Source: CAD feature listing. Evaluate the final solid. Frame: model axes, mm. Face numbers are marked on the shaded views. A direction names the side the tool comes from. Give positions to 0.01 mm unless a question says otherwise; leave off trailing zeros. Write each loop counter-clockwise with the first axis right and the second up, starting at its lowest first coordinate (ties: lowest second). Pieces come first, ordered by that corner, then holes. Notation, with made-up numbers: M 20.25,-10 L 34.25,-10 A19 cw 34.25,10 Z; hole C -10,78.5 d9. An arc over 180 degrees is marked long. Return JSON: item names as keys, results as strings.
Autodesk Inventor part; units mm, degrees
ref_plane "YZ Plane" through (0, 0, 0) normal (1, 0, 0) x (0, 1, 0)
ref_plane "XZ Plane" through (0, 0, 0) normal (0, 1, 0) x (-1, 0, 0)
ref_plane "XY Plane" through (0, 0, 0) normal (0, 0, 1) x (1, 0, 0)
sketch "Sketch1" plane through (0, 0, 0) normal (0, 1, 0) x (-1, 0, 0)
  point P0 (0, 0)
sketch "Sketch2" plane through (0, 0, 0) normal (0, 1, 0) x (-1, 0, 0)
  line L0 (68, -12) -> (68, -66)
  line L1 (68, -66) -> (0, -66)
  line L2 (0, -66) -> (0, -12)
  line L3 (68, -12) -> (0, -12)
  point P0 (0, 0)
  dimension "d0" = 68
  dimension "d138" = 54
extrude "Extrusion1" add sketch "Sketch2" along normal blind 14
sketch "Sketch3" plane through (0, 14, 0) normal (0, 1, 0) x (1, 0, 0)
  point P0 (-68, 66)
sketch "Sketch4" plane through (0, 14, 0) normal (0, 1, 0) x (1, 0, 0)
  line L0 (0, 66) -> (-68, 66)
  line L1 (-30.4814, 66) -> (-28.4814, 66)
  line L2 (-28.4814, 66) -> (-28.4814, 64)
  line L3 (-68, 66) -> (-68, 12)
  line L4 (-68, 37.8423) -> (-68, 39.8423)
  line L5 (-68, 39.8423) -> (-66, 39.8423)
  line L6 (0, 38.8423) -> (0, 36.8423)
  line L7 (0, 36.8423) -> (-2, 36.8423)
  line L8 (-66, 64) -> (-2, 64)
  line L9 (-2, 64) -> (-2, 14)
  line L10 (-2, 14) -> (-66, 14)
  line L11 (-66, 14) -> (-66, 64)
  dimension "d5" = 2
  dimension "d6" = 2
  dimension "d7" = 2
  dimension "d11" = 2
  dimension "d75" = 2
  dimension "d132" = 50
  dimension "d133" = 64
extrude "Extrusion2" cut sketch "Sketch4" against normal blind 13 contours L8 L9 L10 L11
sketch "Sketch7" plane through (0, 14, 0) normal (0, 1, 0) x (1, 0, 0)
  line L0 (-68, 66) -> (-67, 66)
  line L1 (-68, 66) -> (-6, 66)
  line L2 (-68, 65) -> (-68, 66)
  line L3 (0, 66) -> (-7, 66)
  line L4 (-67, 65) -> (-1, 65)
  line L5 (0, 66) -> (-68, 66)
  line L6 (-68, 66) -> (0, 66)
  line L7 (0, 12) -> (0, 66)
  line L8 (0, 12) -> (-1, 12)
  line L9 (-1, 66) -> (0, 66)
  line L10 (0, 66) -> (0, 12)
  line L11 (0, 12) -> (-1, 12)
  line L12 (-68, 12) -> (0, 12)
  line L13 (-1, 65) -> (-1, 12)
  line L14 (0, 12) -> (-1, 12)
  line L15 (-67, 65) -> (-67, 12)
  line L16 (-68, 66) -> (-68, 12)
  line L17 (-67, 12) -> (-68, 12)
  line L18 (-68, 12) -> (-68, 66)
  dimension "d76" = 1
  dimension "d139" = 1
  dimension "d140" = 1
extrude "Extrusion3" cut sketch "Sketch7" against normal blind 2 contours L0 L1 L3 L7 L8 L13 L4 L15 L12 L16 L2
sketch "Sketch8" plane through (0, 14, 0) normal (0, 1, 0) x (1, 0, 0)
  line L0 (0, 12) -> (0, 13)
  line L1 (0, 13) -> (-68, 13)
  line L2 (0, 12) -> (-68, 12)
  line L3 (-68, 12) -> (-68, 13)
  line L4 (-67, 12) -> (-1, 12)
  point P0 (0, 0)
  point P1 (-70, 0)
  dimension "d46" = 68
  dimension "d141" = 1
extrude "Extrusion4" cut sketch "Sketch8" against normal blind 2
sketch "Sketch10" plane through (0, 1, 0) normal (0, 1, 0) x (1, 0, 0)
  line L0 (-31, 2) -> (-41, 2)
  line L1 (-63, 64) -> (-48, 64)
  line L2 (-48, 64) -> (-48, 61)
  line L3 (-48, 61) -> (-63, 61)
  line L4 (-63, 61) -> (-63, 64)
  line L5 (-22, 14) -> (-7, 14)
  line L6 (-7, 14) -> (-7, 17)
  line L7 (-7, 17) -> (-22, 17)
  line L8 (-22, 17) -> (-22, 14)
  line L9 (-66, 14) -> (-66, 64)
  line L10 (-2, 14) -> (-66, 14)
  line L11 (-66, 64) -> (-2, 64)
  line L12 (-2, 64) -> (-2, 14)
  line L13 (-2, 14) -> (-66, 14)
  line L14 (-66, 14) -> (-66, 64)
  point P0 (0, 0)
  point P1 (-21, 64)
  dimension "d57" = 15
  dimension "d58" = 3
  dimension "d61" = 15
  dimension "d79" = 3
extrude "Extrusion5" add sketch "Sketch10" along normal blind 15.5 contours L1 L2 L3 L4 | L8 L7 L6 L5
sketch "Sketch11" plane through (0, 0, 0) normal (0, -1, 0) x (1, 0, 0)
  circle A0 centre (-12, -42.73) radius 4
  circle A1 centre (-33.5, -54.23) radius 1.5
  line L0 (0, 0) -> (0, -66)
  line L1 (0, -66) -> (-68, -66)
  line L2 (-2, -64) -> (-2, -14)
  dimension "d85" = 23.27
  dimension "d86" = 21.5
  dimension "d88" = 8
  dimension "d89" = 3
  dimension "d119" = 11.5
  dimension "d120" = 10
extrude "Extrusion6" cut sketch "Sketch11" against normal blind 9
sketch "Sketch12" plane through (0, 0, 0) normal (0, -1, 0) x (1, 0, 0)
  line L0 (-68, -12) -> (-68, -66)
  line L1 (0, -12) -> (0, -8)
  line L2 (0, -8) -> (-68, -8)
  line L3 (-68, -12) -> (0, -12)
  line L4 (0, -12) -> (-68, -12)
  line L5 (-68, -66) -> (-68, -12)
  line L6 (-68, -66) -> (-72, -66)
  line L7 (-68, -12) -> (-68, -66)
  line L8 (-72, -66) -> (-72, -12)
  line L9 (-68, -8) -> (-72, -8)
  line L10 (-72, -8) -> (-72, -12.2471)
  point P0 (0, 0)
  point P1 (-70, 0)
  dimension "d81" = 4
  dimension "d144" = 0
extrude "Extrusion7" add sketch "Sketch12" against normal blind 24.5
sketch "Sketch15" plane through (0, 0, -66) normal (1, 0, 0) x (0, 0, -1)
  line L0 (-27.77, 14) -> (-18.77, 14)
  line L1 (-18.77, 14) -> (-18.77, 9)
  line L2 (-18.77, 9) -> (-27.77, 9)
  line L3 (-27.77, 9) -> (-27.77, 14)
  line L4 (-54, 0) -> (-54, 24.5)
  line L5 (0, 0) -> (0, 12)
  line L6 (0, 0) -> (-58, 0)
  line L7 (0, 12) -> (-54, 12)
  line L8 (-23.27, -7.8454) -> (-23.27, 0)
  line L9 (-23.27, 0) -> (-23.27, 12)
  line L10 (-53, 14) -> (-1, 14)
  point P0 (-66, 0)
  point P1 (-66, 14.75)
  point P2 (0, 16.75)
  point P3 (-1, 14)
  dimension "d108" = 9
  dimension "d109" = 5
  dimension "d111" = 27.77
  dimension "d174" = 0
extrude "Extrusion9" cut sketch "Sketch15" against normal blind 10 contours L0 L1 L7 L3 | L7 L9 L2 L3 | L1 L2 L9 L7
fillet "Fillet7" radius 3 1 edges at (0, 6, -66)
fillet "Fillet9" radius 3 1 edges at (0, 12.25, -8)
sketch "Sketch17" plane through (-3, 0, -66) normal (0, 0, -1) x (-1, 0, 0)
  line L0 (2, 17) -> (10.5, 17)
  line L1 (10.5, 17) -> (10.5, 12)
  line L2 (10.5, 12) -> (2, 12)
  line L3 (2, 12) -> (2, 17)
  line L4 (17.1, 17) -> (25.6, 17)
  line L5 (25.6, 17) -> (25.6, 12)
  line L6 (25.6, 12) -> (17.1, 12)
  line L7 (17.1, 12) -> (17.1, 17)
  line L8 (66, 0) -> (66, 10.5)
  line L9 (-2, 14) -> (64, 14)
  line L10 (65, 12) -> (0, 12)
  line L11 (-3, 12) -> (-3, 0)
  point P0 (64, 10.5)
  point P1 (0, 12)
  dimension "d151" = 8.5
  dimension "d152" = 8.5
  dimension "d153" = 5
  dimension "d157" = 0
  dimension "d158" = 13.5
  dimension "d160" = 28.6
extrude "Extrusion11" cut sketch "Sketch17" against normal blind 10 contours L0 L1 L9 L3 | L9 L1 L2 L3 | L9 L5 L6 L7 | L7 L4 L5 L9
sketch "Sketch18" plane through (0, 1, 0) normal (0, 1, 0) x (1, 0, 0)
  circle A0 centre (-12, 42.73) radius 4
  line L0 (-12, 38.73) -> (-8, 38.73)
  line L1 (-8, 38.73) -> (-8, 46.73)
  line L2 (-8, 46.73) -> (-16, 46.73)
  line L3 (-16, 46.73) -> (-16, 38.73)
  line L4 (-16, 38.73) -> (-12, 38.73)
  point P0 (0, 0)
  dimension "d169" = 4
  dimension "d170" = 8
  dimension "d171" = 8
extrude "Extrusion12" cut sketch "Sketch18" against normal blind 1
sketch "Sketch19" plane through (-72, 0, -8) normal (0, 0, 1) x (1, 0, 0)
  line L0 (0, 24.5) -> (69, 24.5)
  line L1 (69, 0) -> (0, 0)
  line L2 (0, 24.5) -> (0, 0)
  line L3 (0, 0) -> (0, 24.5)
  line L4 (0, 12.25) -> (70, 12.25)
  line L5 (4, 12) -> (69, 12)
  line L6 (72, 12) -> (72, 0)
  line L7 (0, 0) -> (72, 0)
  line L8 (0, 4.6147) -> (36, 4.6147)
  line L9 (36, 4.6147) -> (36, 24.5)
  line L10 (72, 24.5) -> (4, 24.5)
  circle A0 centre (36, 12.25) radius 2.5
  dimension "d177" = 36
  dimension "d178" = 5
extrude "Extrusion13" cut sketch "Sketch19" against normal blind 4 contours A0 L9 L4 | L4 L9 L5 A0 | A0 L4 L9 | L4 A0 L5 L9 | L5 L9 A0 | L9 L5 A0
sketch "Sketch20" plane through (-72, 0, -66) normal (-1, 0, 0) x (0, 0, 1)
  line L0 (0, 0) -> (0, 24.5)
  line L1 (0, 12.25) -> (58, 12.25)
  line L2 (58, 24.5) -> (58, 0)
  line L3 (3, 0) -> (55, 0)
  line L4 (29, 0) -> (29, 24.5)
  line L5 (54, 24.5) -> (0, 24.5)
  circle A0 centre (29, 12.25) radius 2.5
  point P0 (66, 0)
  dimension "d181" = 5
extrude "Extrusion14" cut sketch "Sketch20" against normal blind 4 contours A0 L4 L1 | L1 L4 A0 | L4 A0 L1 | L1 A0 L4
fillet "Fillet12" radius 3 1 edges at (-72, 12.25, -8)
fillet "Fillet13" radius 3 1 edges at (-72, 12.25, -66)
properties part number "Shell 5 top"
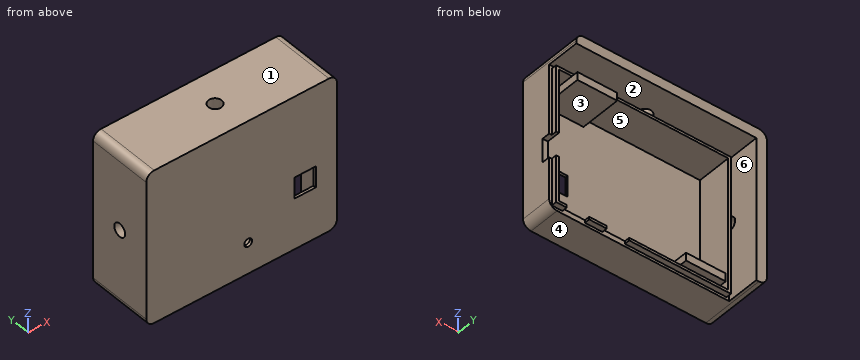
1) Draft query along Z for the marked faces 4, 5 and 6. Return one class per face: released by +Z, released by -Z, zero draft, split by the parting line, or undercut.
Numbers:
{"face 4": "released by -Z", "face 5": "undercut", "face 6": "zero draft"}
2) Line query: line 1 (X direction, y = 13.5, z = -28); line 2 (Z direction, x = -65, y = 6.25); line 3 (X direction, y = 10.75, z = -63). Output: solid intervals per line, ascending. Write a range as [from, to].
Numbers:
{"line 1": "x = [-72, -68], [-67, -66], [-2, -1]", "line 2": "z = [-66, -64], [-14, -8]", "line 3": "x = [-72, -66], [-63, -48], [-2, 0]"}
3) Set-up query: the marked faces 1, 2 and 3. Return all of +Z, -Z, +X, -X, +Y, -Y with unobstructed straight access to the full face (end or side cutting, diameter ignored); none if empty.
Numbers:
{"face 1": "+Z, +X, -X, +Y, -Y", "face 2": "+X, +Y", "face 3": "+Y"}
4) Cut plane A-A, the plane x = -36. Return the cut outline in (y, z), then the cut area to 3 significant figures.
Numbers:
{"outline": "M 0,-66 L 12,-66 L 12,-65 L 14,-65 L 14,-64 L 1,-64 L 1,-14 L 14,-14 L 14,-13 L 12,-13 L 12,-12 L 9.75,-12 L 9.75,-8 L 0,-8 Z; M 14.75,-12 L 24.5,-12 L 24.5,-8 L 14.75,-8 Z", "area": "180 mm²"}
5) Cut plane B-B, the plane z = -54.23. Return the cut outline in (x, y), then the cut area to 3 significant figures.
Numbers:
{"outline": "M -72,0 L -35,0 L -35,1 L -66,1 L -66,14 L -67,14 L -67,12 L -68,12 L -68,24.5 L -72,24.5 Z; M -32,0 L 0,0 L 0,12 L -1,12 L -1,14 L -2,14 L -2,1 L -32,1 Z", "area": "211 mm²"}
6) Cut plane C-C, the plane y = 4.75. Return the cut outline in (x, z), then the cut area to 3 significant figures.
Numbers:
{"outline": "M -72,-63 A3 ccw -69,-66 L -3,-66 A3 ccw 0,-63 L 0,-11 A3 ccw -3,-8 L -69,-8 A3 ccw -72,-11 Z; hole M -66,-64 L -63,-64 L -63,-61 L -48,-61 L -48,-64 L -2,-64 L -2,-14 L -7,-14 L -7,-17 L -22,-17 L -22,-14 L -66,-14 Z", "area": "1,060 mm²"}
7) Contact query for flat-ended pins moving along their axis: pin 1 Ø0.6 at (x, y) = (-0.5, 10.5) entering from -Z; pin 2 Ø0.9 at (x, z) = (-14.5, -15) entering from +Y; pin 3 Ø1 at (x, z) = (-0.5, -42) entering from +Y; pin 4 Ø8 at (y, z) = (12.5, -29) entering from +X. Output: stop coordinate, or through.
Numbers:
{"pin 1": "stops at z = -65.04", "pin 2": "stops at y = 16.5", "pin 3": "stops at y = 9", "pin 4": "stops at x = 0"}
8) Cut plane D-D, the plane z = -23. Return the cut outline in (x, y), then the cut area to 3 significant figures.
Numbers:
{"outline": "M -72,0 L 0,0 L 0,12 L -1,12 L -1,14 L -2,14 L -2,1 L -66,1 L -66,14 L -67,14 L -67,12 L -68,12 L -68,24.5 L -72,24.5 Z", "area": "214 mm²"}
